Solid Edge part; units mm, degrees
sketch "Sketch1" plane through (0, 0, 0) normal (0, 0, 1) x (1, 0, 0)
  circle A0 centre (0, 0) radius 34.56
  circle A1 centre (0, 0) radius 26
extrude "Protrusion1" add sketch "Sketch1" along normal blind 7.2
sketch "Sketch2" plane through (0, 0, 0) normal (0, 0, -1) x (-1, 0, 0)
  circle A0 centre (0, 29) radius 2.65
extrude "Hål_för_skruv" cut sketch "Sketch2" along normal mid plane 493.3012
pattern_circular "Pattern1" count 6 over 360 about axis through (0, 0, 0) along (0, 0, 1) of "Hål_för_skruv"
properties material "Steel"
Input: part model. Units: mm. Frame: model coordinates. Give positions to 0.01 mm unless a question says otherwise; leave off trailing zeros. Order: outer loops, then holes, each group sorted by start corner. A loop starts at its lowest first (then second) coordinate and runs counter-clockwise, first axis right, second up. Notation, with made-up numbers: (54, -16.5) - (95, -16.5) arc R23 cw to (95, 0.5) - close; hole circle Ø3 at (-28, 81.25). An arc over 180 degrees is marked (long way). Use a Markdown table: item, result.
(1) Section query B-B (x = 0). Output: boundary loops of the cut face in (y, z).
Computed values:
| item | result |
|---|---|
| outline | (-34.56, 0) - (-31.65, 0) - (-31.65, 7.2) - (-34.56, 7.2) - close; (-26.35, 0) - (-26, 0) - (-26, 7.2) - (-26.35, 7.2) - close; (26, 0) - (26.35, 0) - (26.35, 7.2) - (26, 7.2) - close; (31.65, 0) - (34.56, 0) - (34.56, 7.2) - (31.65, 7.2) - close |
(2) Pin query (flat end, axial travel): pin 1 (4 mm diameter, centred on x = 0, y = 29, fed in from -Z); pin 2 (4 mm diameter, centred on x = 3.5, z = 4, fed in from +Y); pin 3 (3 mm diameter, centred on x = 23, z = 2, fed in from +Y); pin 4 (2 mm diameter, centred on y = 12.5, z = 1, fed in from +X). Return the tip coordinate at first contact, or that it passes through.
Computed values:
| item | result |
|---|---|
| pin 1 | passes through |
| pin 2 | stops at y = 34.53 |
| pin 3 | stops at y = 27.06 |
| pin 4 | stops at x = 32.59 |
(3) Section query A-A (y = 0). Output: boundary loops of the cut face in (x, z).
Computed values:
| item | result |
|---|---|
| outline | (-34.56, 0) - (-26, 0) - (-26, 7.2) - (-34.56, 7.2) - close; (26, 0) - (34.56, 0) - (34.56, 7.2) - (26, 7.2) - close |
(4) Section query D-D (z = 4). Output: boundary loops of the cut face in (x, y), then the cut area to 3 significant figures.
Computed values:
| item | result |
|---|---|
| outline | circle Ø69.12 at (0, 0); hole circle Ø5.3 at (-25.11, -14.5); hole circle Ø5.3 at (-25.11, 14.5); hole circle Ø52 at (0, 0); hole circle Ø5.3 at (0, -29); hole circle Ø5.3 at (0, 29); hole circle Ø5.3 at (25.11, -14.5); hole circle Ø5.3 at (25.11, 14.5) |
| area | 1,500 mm2 |
(5) Draft query along Y for faces 1 (the flat face through (5, 26, 0)), 2 (the cylindrical face through (-27.64, -13.7, 3.55)), 3 (the cylindrical face through (-0.34, -31.63, 3.55)), 4 (the cylindrical face through (32.964, -10.381, 3.55)). Return one class per face: released by +Y, released by -Y, zero draft, split by the parting line, or undercut.
Computed values:
| item | result |
|---|---|
| face 1 | zero draft |
| face 2 | undercut |
| face 3 | undercut |
| face 4 | split by the parting line |
(6) Section query C-C (x = -21.5). Output: boundary loops of the cut face in (y, z).
Computed values:
| item | result |
|---|---|
| outline | (-27.06, 0) - (-14.62, 0) - (-14.62, 7.2) - (-27.06, 7.2) - close; (14.62, 0) - (27.06, 0) - (27.06, 7.2) - (14.62, 7.2) - close |
(7) Line query: line 1 (Y direction, x = 0, z = 5.75); line 2 (Y direction, x = -2, z = 6); line 3 (X direction, y = 22.5, z = 3). Output: solid intervals per line, ascending. Write a range as from..to.
Computed values:
| item | result |
|---|---|
| line 1 | y = -34.56..-31.65, -26.35..-26, 26..26.35, 31.65..34.56 |
| line 2 | y = -34.5..-30.74, -27.26..-25.92, 25.92..27.26, 30.74..34.5 |
| line 3 | x = -26.23..-13.03, 13.03..26.23 |
